```python
from build123d import *

# Parameters (mm, degrees)
BOSS_EXTRUDE1_DEPTH      = 3
BOSS_EXTRUDE1_DEPTH_BACK = 3
SKETCH1_W                = 40.5
SKETCH1_H                = 10.5
SKETCH1_R                = 2.25


with BuildPart() as part:
    # Sketch1 → Boss-Extrude1 (new, two sides: drawn at the far end of the back side and taken through both)
    with BuildSketch(Plane.XY.offset(-BOSS_EXTRUDE1_DEPTH_BACK)):
        Rectangle(SKETCH1_W, SKETCH1_H)
        with Locations((-14.5, 0)):
            Circle(SKETCH1_R, mode=Mode.SUBTRACT)
        with Locations((14.5, 0)):
            Circle(SKETCH1_R, mode=Mode.SUBTRACT)
    extrude(amount=BOSS_EXTRUDE1_DEPTH + BOSS_EXTRUDE1_DEPTH_BACK)


solid = part.part
```
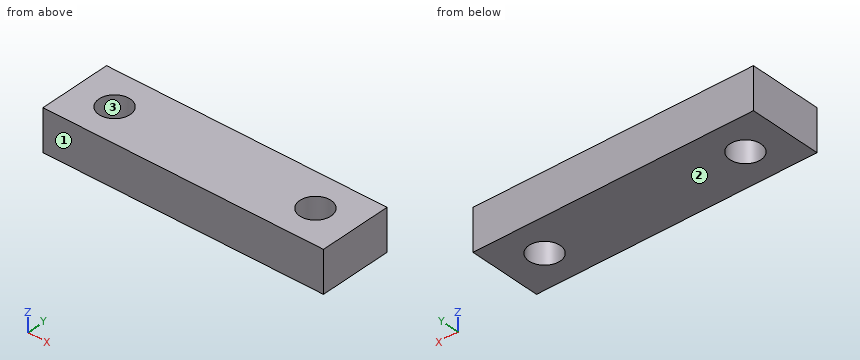
Verification items for the finished model (mm, model axes). Face numbers are marked on the shaded views. Coordinates: 2 decimals unless noted, no trailing zeros. Write each loop counter-clockwise with the first axis right and the second up, starting at its lowest first coordinate (ties: lowest second). Pieces come first, ordered by that corner, then holes. Notation, with made-up numbers: M -22.5,74.25 L 16.5,74.25 A13 ccw 16.5,81.25 Z; hole C 62.5,-34 d10. An arc over 180 degrees is marked long. Answer as a JSON object with one key per item and string values. Group by question number.
(1) Material ranges on line 1 (X direction, y = 2, z = 0.5); line 2 (Y direction, x = -14.5, z = 0.55); line 3 (X direction, y = 0.5, z = -0.5), recorded low to high.
(2) Cross-section at B-B, the plane x = -14.5. Record the cut outline in (y, z).
(3) Release check for a two-part mould opening along Y. For the marked faces 1, 2 and 3 record: +Y half, -Y half, draft (parallel to the pull), parting line (faces both ways), or undercut.
(4) Cross-section at A-A, the plane y = 0. Record the cut outline in (x, z).
(5) Cross-section at C-C, the plane z = -2.15. Record the cut outline in (x, y).
Reply:
{
 "1": {"line 1": "-20.25 to -15.53, -13.47 to 13.47, 15.53 to 20.25", "line 2": "-5.25 to -2.25, 2.25 to 5.25", "line 3": "-20.25 to -16.69, -12.31 to 12.31, 16.69 to 20.25"},
 "2": {"outline": "M -5.25,-3 L -2.25,-3 L -2.25,3 L -5.25,3 Z; M 2.25,-3 L 5.25,-3 L 5.25,3 L 2.25,3 Z"},
 "3": {"face 1": "-Y half", "face 2": "draft", "face 3": "undercut"},
 "4": {"outline": "M -20.25,-3 L -16.75,-3 L -16.75,3 L -20.25,3 Z; M -12.25,-3 L 12.25,-3 L 12.25,3 L -12.25,3 Z; M 16.75,-3 L 20.25,-3 L 20.25,3 L 16.75,3 Z"},
 "5": {"outline": "M -20.25,-5.25 L 20.25,-5.25 L 20.25,5.25 L -20.25,5.25 Z; hole C -14.5,0 d4.5; hole C 14.5,0 d4.5"}
}
